Build history of the part. All positions in model axes, mm. Face numbers are marked on the shaded views. A direction names the side the tool comes from. Give positions to 0.01 mm unless a question says otherwise; leave off trailing zeros. Order: outer loops, then holes, each group sorted by start corner. A loop starts at its lowest first (then second) coordinate and runs counter-clockwise, first axis right, second up. Notation, with made-up numbers: (53.25, 1) - (88.25, 1) arc R32 ccw to (88.25, 34) - close; hole circle Ø1 at (36, 18). An arc over 180 degrees is marked (long way). Write each question's results on one line, items separated by ' | '. Start each with the question number.
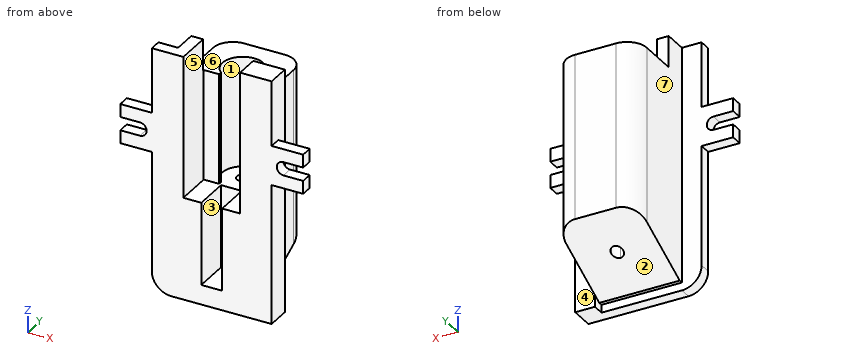
from build123d import *

# Parameters (mm, degrees)
SKETCH1_W           = 4.55
SKETCH1_H           = 21
BOSS_EXTRUDE1_DEPTH = 3
FILLET1_R           = 5
BOSS_EXTRUDE2_DEPTH = 6
SKETCH9_W           = 20.4
SKETCH9_H           = 52
BOSS_EXTRUDE4_DEPTH = 15
CHAMFER4_SIZE       = 20
CHAMFER4_SIZE2      = 10
FILLET5_R           = 5
CUT_EXTRUDE6_DEPTH  = 28
CUT_EXTRUDE7_DEPTH  = 64.484171256
SKETCH16_W          = 32
SKETCH16_H          = 3.3
CUT_EXTRUDE8_DEPTH  = 3
SKETCH17_W          = 5
SKETCH17_H          = 62
BOSS_EXTRUDE5_DEPTH = 3


with BuildPart() as part:
    # Sketch1 → Boss-Extrude1 (new body)
    with BuildSketch(Plane(origin=(0, 0, 0), x_dir=(1, 0, 0), z_dir=(0, 1, 0))):
        with BuildLine():
            Line((-15.2, -14.5), (-15.2, -31))
            Line((-15.2, -31), (-7.2, -31))
            Line((-7.2, -31), (-7.2, 5))
            Line((-7.2, 5), (-7.2, 26))
            Line((-7.2, 26), (-2.65, 26))
            Line((-2.65, 26), (2.65, 26))
            Line((2.65, 26), (7.2, 26))
            Line((7.2, 26), (7.2, 5))
            Line((7.2, 5), (7.2, -31))
            Line((7.2, -31), (15.2, -31))
            Line((15.2, -31), (15.2, -14.5))
            Line((15.2, -14.5), (23.2, -14.5))
            Line((23.2, -14.5), (23.2, -11.2))
            Line((23.2, -11.2), (18.2, -11.2))
            ThreePointArc((18.2, -11.2), (16.5, -9.5), (18.2, -7.8))
            Line((18.2, -7.8), (23.2, -7.8))
            Line((23.2, -7.8), (23.2, -4.5))
            Line((23.2, -4.5), (15.2, -4.5))
            Line((15.2, -4.5), (15.2, 31))
            Line((15.2, 31), (-15.2, 31))
            Line((-15.2, 31), (-15.2, -4.5))
            Line((-15.2, -4.5), (-23.2, -4.5))
            Line((-23.2, -4.5), (-23.2, -7.8))
            Line((-23.2, -7.8), (-18.2, -7.8))
            ThreePointArc((-18.2, -7.8), (-16.5, -9.5), (-18.2, -11.2))
            Line((-18.2, -11.2), (-23.2, -11.2))
            Line((-23.2, -11.2), (-23.2, -14.5))
            Line((-23.2, -14.5), (-15.2, -14.5))
        make_face()
        with Locations((-4.925, 15.5)):
            Rectangle(SKETCH1_W, SKETCH1_H)
        with Locations((4.925, 15.5)):
            Rectangle(SKETCH1_W, SKETCH1_H)
    extrude(amount=BOSS_EXTRUDE1_DEPTH)

    # Fillet1
    fillet1_edges = [part.edges().sort_by_distance(p)[0] for p in [
        (-15.2, 1.5, -31),
    ]]
    fillet(fillet1_edges, radius=FILLET1_R)

    # Sketch3 → Boss-Extrude2 (add)
    with BuildSketch(Plane(origin=(0, 3, 0), x_dir=(1, 0, 0), z_dir=(0, 1, 0))):
        Polygon((10.2, 29), (-10.2, 29), (-10.2, -31), (-7.2, -31), (-7.2, 5), (-2.65, 5), (-2.65, 26), (2.65, 26), (2.65, 5), (7.2, 5), (7.2, -31), (10.2, -31), align=None)
    extrude(amount=BOSS_EXTRUDE2_DEPTH)

    # Sketch9 → Boss-Extrude4 (add)
    with BuildSketch(Plane(origin=(0, 9, 0), x_dir=(1, 0, 0), z_dir=(0, 1, 0))):
        with Locations((0, 3)):
            Rectangle(SKETCH9_W, SKETCH9_H)
    extrude(amount=BOSS_EXTRUDE4_DEPTH)

    # Chamfer4
    chamfer4_edges = [part.edges().sort_by_distance(p)[0] for p in [
        (0, 24, -29),
    ]]
    chamfer4_side = [part.faces().sort_by_distance(p)[0] for p in [
        (0, 13.5, -29),
    ]]
    chamfer(chamfer4_edges, length=CHAMFER4_SIZE, length2=CHAMFER4_SIZE2, reference=chamfer4_side[0])

    # Fillet5
    fillet5_edges = [part.edges().sort_by_distance(p)[0] for p in [
        (10.2, 24, 2),
        (-10.2, 24, 2),
    ]]
    fillet(fillet5_edges, radius=FILLET5_R)

    # Sketch15 → Cut-Extrude6 (cut)
    with BuildSketch(Plane.XY.offset(23)):
        with BuildLine():
            Line((7.2, 9), (7.2, 9.3))
            Line((7.2, 9.3), (3.304542328, 9.3))
            Line((3.304542328, 9.3), (3.304542328, 10.2))
            ThreePointArc((3.304542328, 10.2), (0, 19.3), (-3.304542328, 10.2))
            Line((-3.304542328, 10.2), (-3.304542328, 9.3))
            Line((-3.304542328, 9.3), (-7.2, 9.3))
            Line((-7.2, 9.3), (-7.2, 9))
            Line((-7.2, 9), (7.2, 9))
        make_face()
    extrude(amount=-CUT_EXTRUDE6_DEPTH, mode=Mode.SUBTRACT)

    # Sketch15<6> → Cut-Extrude7 (cut, through all)
    with BuildSketch(Plane.XY.offset(23)):
        with BuildLine():
            ThreePointArc((0, 15.65), (-1.5, 14.15), (0, 12.65))
            Line((0, 12.65), (0, 15.65))
        make_face()
        with BuildLine():
            Line((0, 15.65), (0, 12.65))
            ThreePointArc((0, 12.65), (1.060660172, 13.089339828), (1.5, 14.15))
            ThreePointArc((1.5, 14.15), (1.060660172, 15.210660172), (0, 15.65))
        make_face()
    extrude(amount=-CUT_EXTRUDE7_DEPTH, mode=Mode.SUBTRACT)

    # Sketch16 → Cut-Extrude8 (cut)
    with BuildSketch(Plane(origin=(10.2, 0, 0), x_dir=(0, 0, -1), z_dir=(1, 0, 0))):
        with Locations((-15, 7.65)):
            Rectangle(SKETCH16_W, SKETCH16_H)
    extrude(amount=-CUT_EXTRUDE8_DEPTH, mode=Mode.SUBTRACT)

    # Sketch17 → Boss-Extrude5 (add)
    with BuildSketch(Plane(origin=(0, 3, 0), x_dir=(1, 0, 0), z_dir=(0, 1, 0))):
        with Locations((12.7, 0)):
            Rectangle(SKETCH17_W, SKETCH17_H)
    extrude(amount=BOSS_EXTRUDE5_DEPTH)


solid = part.part
Item 1: Which spindle directions (+Z, -Z, +X, -X, +Y, -Y) get a long thin tool onto all of the face, cutting with end or side? Do the marked faces 5, 6 and 7. Say none if no direction does.
Item 2: Cut at C-C, the plane y = 18.25. List the corners of the cut face in (x, z) (3 decimals).
Item 3: Probe line 1 along X through (y, z) = (14.15, 10.5); line 2 along X through (y, z) = (4.5, 25); line 3 along X through (y, z) = (12.25, -19). List the from-to ranges inside material, lowest first. Write a range as from..to.
Item 4: Flat gauge pins, fed straight in: pin 1 Ø2.5 at (x, y) = (1, 5) entering from +Z; pin 2 Ø7 at (y, z) = (6, -12) entering from +X; pin 3 Ø6 at (x, y) = (2.5, 20.5) entering from +Z. Where does each tip first touch, or does it go through?
Item 5: Cut at D-D, the plane x = 8.5. List the corners of the cut face in (y, z), then the cut area to 3 significant figures.
Item 6: Cut at A-A, the plane z = 9.5. List the corners of the cut face in (x, y).
Item 7: Cut at B-B, the plane z = -10. List the corners of the cut face in (x, y).
Item 8: Two-plate mould, pull along Y, no slides. Class the marked faces 1, 2, 3 and 4: +Y half, -Y half, draft (parallel to the pull), parting line (faces both ways), or undercut.
Values found:
1) face 5: +Z, -Y | face 6: +Z, +X, -X, +Y | face 7: +Z, -Z, -X, +Y
2) outline: (-10.2, -21.875) - (10.2, -21.875) - (10.2, 23) - (3.116, 23) - (3.116, -5) - (-3.116, -5) - (-3.116, 23) - (-10.2, 23) - close
3) line 1: x = -10.2..-5.15, 5.15..10.2 | line 2: x = -10.2..-7.2, 7.2..15.2 | line 3: x = -10.2..10.2
4) pin 1: stops at z = -26 | pin 2: stops at x = 15.2 | pin 3: stops at z = 23
5) outline: (0, -31) - (3, -31) - (3, -29) - (4, -29) - (22.76, -19.62) - (22.76, 23) - (9.3, 23) - (9.3, -1) - (6, -1) - (6, 31) - (0, 31) - close | area: 1,070 mm2
6) outline: (-16.5, 0) - (-7.2, 0) - (-7.2, 9.3) - (-3.3, 9.3) - (-3.3, 10.2) arc R5.15 cw (long way) to (3.3, 10.2) - (3.3, 9.3) - (10.2, 9.3) - (10.2, 19) arc R5 ccw to (5.2, 24) - (-5.2, 24) arc R5 ccw to (-10.2, 19) - (-10.2, 3) - (-16.5, 3) - close; (7.2, 0) - (16.5, 0) - (16.5, 3) - (15.2, 3) - (15.2, 6) - (7.2, 6) - close
7) outline: (-15.2, 0) - (-2.65, 0) - (-2.65, 9) - (2.65, 9) - (2.65, 0) - (15.2, 0) - (15.2, 6) - (10.2, 6) - (10.2, 19) arc R5 ccw to (5.2, 24) - (-5.2, 24) arc R5 ccw to (-10.2, 19) - (-10.2, 3) - (-15.2, 3) - close; hole circle Ø3 at (0, 14.15)
8) face 1: undercut | face 2: +Y half | face 3: draft | face 4: undercut
